Part model, mm, in its own coordinate system. A direction names the side the tool comes from. Round coordinates to 2 decimals unless told otherwise and drop trailing zeros. Loops run counter-clockwise (first coordinate to the right, second up) from the corner with the lowest first, then second, coordinate; pieces in that order, holes last. Notation, with made-up numbers: M -37,1.5 L -6,1.5 A27 cw -6,36.5 Z; hole C -34,82.25 d5. An arc over 180 degrees is marked long. Put each result on its own line as item: value. Start each with the question number.
1) Pull direction Z, two halves, no side cores. Call faces 6 (the flat face through (-21, 2, 0)), 7 (the flat face through (19, 1, -20)): +Z half, -Z half, draft (parallel to the pull), parting line (faces both ways), or undercut.
2) Slice it at B-B on z = -32. Give the cut face in (x, y) (3 decimals).
3) Slice it at D-D on y = 3.25. State how many separate pieces and enclosed holes the cut face has, then the cut area to 3 significant figures.
4) Which spindle directions (+Z, -Z, +X, -X, +Y, -Y) get a long thin tool onto all of the face, cutting with end or side? Do faces 1 (the flat face through (0, -4, 29.5)), 2 (the flat face through (19, 1, 0)), 3 (the flat face through (5, 3, 32)), 4 (the flat face through (0, -2.4, 32)), 5 (the flat face through (0, 3, -34.5)). Say none if no direction does.
5) Slice it at A-A on y = -1. Give the cut face in (x, z), then the cut area to 3 significant figures.
6) Slice it at C-C on x = -18. Give the cut face in (y, z), then the cut area to 3 significant figures.
7) Probe line 1 along Z through (x, y) = (0, 3.25); line 2 along X through (y, z) = (0.5, 14); line 3 along X through (y, z) = (2.95, 22). List the from-to ranges inside material, lowest first.
8) Drop flat-ended pins along their axis: pin 1 Ø0.5 at (x, z) = (0, 32) entering from +Y; pin 2 Ø6 at (x, z) = (-1, -13) entering from -Y; pin 3 Ø2 at (x, y) = (11.5, 1) entering from +Z. Give the stop position or say it passes through.
```python
from build123d import *

# Parameters (mm, degrees)
F1_DEPTH  = 4
F2_W      = 10
F2_H      = 2.5
F3_DEPTH  = 5.7
F5_DEPTH  = 2.5
F6_R      = 1.5
F7_DEPTH  = 4
F9_DEPTH  = 2
F10_R     = 4.5
F10_R_2   = 1.5
F11_DEPTH = 2
F13_DEPTH = 2
F15_DEPTH = 2
F16_R     = 1.375
F17_DEPTH = 0.8
F18_SIZE  = 2.5
F19_W     = 10
F19_H     = 4.5
F20_DEPTH = 2
F21_R     = 1
F22_R     = 0.5
F23_R     = 0.5


with BuildPart() as f1:
    # F0 (on Front) → F1 (new body)
    with BuildSketch(Plane.XZ):
        Polygon((-14, 29.5), (-21, 29.5), (-21, -29.5), (-14, -29.5), (-5, -39.5), (5, -39.5), (14, -29.5), (21, -29.5), (21, 29.5), (14, 29.5), (5, 39.5), (-5, 39.5), align=None)
    extrude(amount=-F1_DEPTH)

    # F2 (on face) → F3 (join)
    with BuildSketch(Plane.XZ):
        with Locations((0, 38.25)):
            Rectangle(F2_W, F2_H)
        with Locations((0, -38.25)):
            Rectangle(F2_W, F2_H)
    extrude(amount=F3_DEPTH)

    # F4 (on face) → F5 (join)
    with BuildSketch(Plane.XZ.offset(5.7)):
        Polygon((5, 39.5), (-5, 39.5), (-5, 37), (-3.677548, 29.5), (3.677548, 29.5), (5, 37), align=None)
        Polygon((3.677548, -29.5), (-3.677548, -29.5), (-5, -37), (-5, -39.5), (5, -39.5), (5, -37), align=None)
    extrude(amount=-F5_DEPTH)

    # F6 (on face) → F7 (cut, through all)
    with BuildSketch(Plane.XZ):
        with Locations((0, 22)):
            Circle(F6_R)
        with Locations((0, -22)):
            Circle(F6_R)
    extrude(amount=-F7_DEPTH, mode=Mode.SUBTRACT)

    # F8 (on face) → F9 (cut)
    with BuildSketch(Plane.XZ):
        Polygon((-19, -27.5), (-13.109275, -27.5), (-6.359275, -35), (6.359275, -35), (13.109275, -27.5), (19, -27.5), (19, 27.5), (13.109275, 27.5), (6.359275, 35), (-6.359275, 35), (-13.109275, 27.5), (-19, 27.5), align=None)
    extrude(amount=-F9_DEPTH, mode=Mode.SUBTRACT)

    # F10 (on face) → F11 (join, through all)
    with BuildSketch(Plane.XZ.offset(-2)):
        with Locations((0, -22)):
            Circle(F10_R)
        with Locations((0, -22)):
            Circle(F10_R_2, mode=Mode.SUBTRACT)
        with Locations((0, 22)):
            Circle(F10_R)
        with Locations((0, 22)):
            Circle(F10_R_2, mode=Mode.SUBTRACT)
    extrude(amount=F11_DEPTH)

    # F12 (on face) → F13 (cut, through all)
    with BuildSketch(Plane.XZ):
        Polygon((-4.559275, -37), (4.559275, -37), (6.359275, -35), (5, -35), (-5, -35), (-6.359275, -35), align=None)
        Polygon((4.559275, 37), (-4.559275, 37), (-6.359275, 35), (6.359275, 35), align=None)
    extrude(amount=-F13_DEPTH, mode=Mode.SUBTRACT)

    # F14 (on face) → F15 (join, through all)
    with BuildSketch(Plane.XZ.offset(-2)):
        Polygon((5.484828, -12), (19, -12), (19, -10), (7.216878, -10), (1.443376, 0), (7.216878, 10), (19, 10), (19, 12), (5.484828, 12), (0, 2.5), (-5.484828, 12), (-19, 12), (-19, 10), (-7.216878, 10), (-1.443376, 0), (-7.216878, -10), (-19, -10), (-19, -12), (-5.484828, -12), (0, -2.5), align=None)
    extrude(amount=F15_DEPTH)

    # F16 (on face) → F17 (join)
    with BuildSketch(Plane(origin=(0, -3.2, 0), x_dir=(-1, 0, 0), z_dir=(0, 1, 0))):
        with Locations((0, -32)):
            Circle(F16_R)
        with Locations((0, 32)):
            Circle(F16_R)
    extrude(amount=F17_DEPTH)

    # F18
    f18_edges = [f1.edges().sort_by_distance(p)[0] for p in [
        (-1.5, 0, -22),
        (-1.5, 0, 22),
    ]]
    chamfer(f18_edges, length=F18_SIZE)

    # F19 (on face) → F20 (cut, through all)
    with BuildSketch(Plane(origin=(0, 4, 0), x_dir=(-1, 0, 0), z_dir=(0, 1, 0))):
        with Locations((0, 32.25)):
            Rectangle(F19_W, F19_H)
        with Locations((0, -32.25)):
            Rectangle(F19_W, F19_H)
    extrude(amount=-F20_DEPTH, mode=Mode.SUBTRACT)

    # F21
    f21_edges = [f1.edges().sort_by_distance(p)[0] for p in [
        (-5, 3, 34.5),
        (5, 3, 30),
        (5, 3, 34.5),
        (-5, 3, 30),
        (5, 3, -34.5),
        (5, 3, -30),
        (-5, 3, -30),
        (-5, 3, -34.5),
    ]]
    fillet(f21_edges, radius=F21_R)

    # F22
    f22_edges = [f1.edges().sort_by_distance(p)[0] for p in [
        (1.375, -2.4, -32),
        (1.375, -2.4, 32),
    ]]
    fillet(f22_edges, radius=F22_R)

    # F23
    f23_edges = [f1.edges().sort_by_distance(p)[0] for p in [
        (0, 2, 37),
        (0, 2, -37),
        (0, -3.2, 37),
        (0, -3.2, -37),
    ]]
    fillet(f23_edges, radius=F23_R)


solid = f1.part
```
Recorded:
1. face 6: draft
1. face 7: undercut
2. outline: M -11.75,0 L -9.059,0 L -9.059,2 L -5,2 L -5,4 L -11.75,4 Z; M -4.118,-5.7 L 4.118,-5.7 L 4.118,-3.2 L 1.375,-3.2 L 1.375,-2.9 A0.5 ccw 0.875,-2.4 L -0.875,-2.4 A0.5 ccw -1.375,-2.9 L -1.375,-3.2 L -4.118,-3.2 Z; M 5,2 L 9.059,2 L 9.059,0 L 11.75,0 L 11.75,4 L 5,4 Z
3. separate pieces: 1
3. enclosed holes: 4
3. area: 2,760 mm2
4. face 1: +X, -X, -Y
4. face 2: -Y
4. face 3: +Y, -Y
4. face 4: +X, -X, +Y
4. face 5: +Y
5. outline: M -5,-39.5 L 5,-39.5 L 5,-37 L -5,-37 Z; M -5,37 L 5,37 L 5,39.5 L -5,39.5 Z
5. area: 50.0 mm2
6. outline: M 0,-29.5 L 4,-29.5 L 4,29.5 L 0,29.5 L 0,27.5 L 2,27.5 L 2,12 L 0,12 L 0,10 L 2,10 L 2,-10 L 0,-10 L 0,-12 L 2,-12 L 2,-27.5 L 0,-27.5 Z
6. area: 134 mm2
7. line 1: z = -39.5 to -34.5, -30 to -23.5, -20.5 to 20.5, 23.5 to 30, 34.5 to 39.5
7. line 2: x = -21 to -19, 19 to 21
7. line 3: x = -21 to -1.5, 1.5 to 21
8. pin 1: stops at y = -2.4
8. pin 2: stops at y = 2
8. pin 3: stops at z = 33.39
